Part model, mm, in its own coordinate system. A direction names the side the tool comes from. Coordinates: 2 decimals unless noted, no trailing zeros. Write each loop counter-clockwise with the first axis right and the second up, starting at its lowest first coordinate (ties: lowest second). Pieces come first, ordered by that corner, then holes. Notation, with made-up numbers: M 83.5,-4.75 L 116.5,-4.75 A20 ccw 116.5,17.25 Z; hole C 53.5,68 d2. An arc over 180 degrees is marked long. Use a Markdown table: item, result. Add a question column.
Q1. Wall check: L1, parallel to Y at x = -19, z = 4.5; L2, parallel to X at y = 15, z = 13; L3, parallel to X at y = -6.5, z = 1.25. Give the ranges that are in metal, low to high. Write a range as from..to.
Q2. Slice it at C-C on y = 5.5. Write the cut outline in (x, z), then the cut area to 3 significant figures.
Q3. Slice it at A-A on z = 12.5. Write the cut outline in (x, y).
Q4. Slice it at D-D on z = 3. Write the cut outline in (x, y).
Q5. Pin check, flat tips, straight feed: pin 1 Ø11 at (x, z) = (-0.5, 16) entering from +Y; pin 2 Ø1.5 at (y, z) = (13.5, 13.5) entering from -X; pin 3 Ø0.6 at (x, z) = (-7.5, 23) entering from -Y. Stop position of each tip, or through.
Q6. Slice it at B-B on x = 2. Write the cut outline in (y, z), then the cut area to 3 significant figures.
Q7. Tool access for faces 5 (the flat face through (-1, -10.25, 6)), 6 (the flat face through (-45.75, -6.9, 22.5)), 7 (the flat face through (41.75, 13, 11)), 8 (the flat face through (-8, 12.25, 13)): list every direction of +Z, -Z, +X, -X, +Y, -Y with a clear straight run to the whole face (end or side of a thin tool).
Q8. Mould opens along Y. For faces 1 (the flat face through (-5, 10.25, 11)), 2 (the flat face through (38.75, 13, 11)), 3 (the flat face through (22, 17.25, 1)), 4 (the flat face through (-2, 7.25, 23)) say: released by +Y, released by -Y, zero draft, split by the parting line, or undercut.
from build123d import *

# Parameters (mm, degrees)
EXTRUDE_1_DEPTH          = 8
EXTRUDE_3_DEPTH          = 14
CUT_EXTRUDE_1_DEPTH      = 55.485089704
CUT_EXTRUDE_1_DEPTH_BACK = 55.485089704
SKETCH_4_W               = 2
SKETCH_4_H               = 24.5
SKETCH_7_W               = 2
SKETCH_7_H               = 2
SKETCH_7_W_2             = 5
EXTRUDE_6_DEPTH          = 14
EXTRUDE_4_DEPTH          = 2
SKETCH_8_W               = 85.5
SKETCH_8_H               = 1.5
EXTRUDE_7_DEPTH          = 5


with BuildPart() as part:
    # Эскиз1 → Бобышка-Вытянуть1 (new body)
    with BuildSketch(Plane.XY):
        Polygon((47.75, 12.25), (44.75, 12.25), (44.75, 17.25), (35.75, 17.25), (35.75, 12.25), (-49.75, 12.25), (-49.75, -12.25), (47.75, -12.25), (47.75, -10.25), (-47.75, -10.25), (-47.75, 10.25), (38.75, 10.25), (38.75, 15.25), (41.75, 15.25), (41.75, 12.25), (41.75, 10.25), (47.75, 10.25), align=None)
    extrude(amount=EXTRUDE_1_DEPTH)

    # Эскиз2 → Бобышка-Вытянуть3 (add)
    with BuildSketch(Plane.XY.offset(8)):
        Polygon((44.75, 10.25), (47.75, 10.25), (47.75, 12.25), (44.75, 12.25), (44.75, 15.25), (44.75, 17.25), (41.75, 17.25), (35.75, 17.25), (35.75, 15.25), (35.75, 12.25), (-47.75, 12.25), (-49.75, 12.25), (-49.75, 10.25), (-49.75, -10.25), (-49.75, -12.25), (-47.75, -12.25), (-47.75, -10.25), (-47.75, 10.25), (35.75, 10.25), (38.75, 10.25), (38.75, 12.25), (38.75, 15.25), (41.75, 15.25), (41.75, 10.25), align=None)
    extrude(amount=EXTRUDE_3_DEPTH)

    # Эскиз4 → Вырез-Вытянуть1 (cut, two sides: drawn at the far end of the back side and taken through both)
    with BuildSketch(Plane.XY.offset(8).offset(-CUT_EXTRUDE_1_DEPTH_BACK)):
        with Locations((46.75, 0)):
            Rectangle(SKETCH_4_W, SKETCH_4_H)
    extrude(amount=CUT_EXTRUDE_1_DEPTH + CUT_EXTRUDE_1_DEPTH_BACK, mode=Mode.SUBTRACT)

    # Эскиз7 → Бобышка-Вытянуть6 (add)
    with BuildSketch(Plane.XY.offset(8)):
        with Locations((-46.75, -11.25)):
            Rectangle(SKETCH_7_W, SKETCH_7_H)
        with Locations((43.25, -11.25)):
            Rectangle(SKETCH_7_W_2, SKETCH_7_H)
    extrude(amount=EXTRUDE_6_DEPTH)

    # Эскиз5 → Бобышка-Вытянуть4 (add)
    with BuildSketch(Plane.XY.offset(22)):
        Polygon((45.75, -12.25), (40.75, -12.25), (40.75, 7.25), (-45.75, 7.25), (-45.75, -12.25), (-49.75, -12.25), (-49.75, 12.25), (35.75, 12.25), (35.75, 17.25), (44.75, 17.25), (44.75, 12.25), (45.75, 12.25), align=None)
    extrude(amount=EXTRUDE_4_DEPTH)

    # Эскиз8 → Бобышка-Вытянуть7 (add)
    with BuildSketch(Plane(origin=(0, 12.25, 0), x_dir=(1, 0, 0), z_dir=(0, 1, 0))):
        with Locations((-7, -0.75)):
            Rectangle(SKETCH_8_W, SKETCH_8_H)
    extrude(amount=EXTRUDE_7_DEPTH)


solid = part.part
Recorded:
| question | item | result |
|---|---|---|
| 1 | L1 | -12.25..-10.25, 10.25..12.25 |
| 1 | L2 | 35.75..38.75, 41.75..44.75 |
| 1 | L3 | -49.75..-47.75 |
| 2 | outline | M -49.75,0 L -47.75,0 L -47.75,22 L -45.75,22 L -45.75,24 L -49.75,24 Z; M 40.75,22 L 45.75,22 L 45.75,24 L 40.75,24 Z |
| 2 | area | 62.0 mm² |
| 3 | outline | M -49.75,-12.25 L -45.75,-12.25 L -45.75,-10.25 L -47.75,-10.25 L -47.75,10.25 L 38.75,10.25 L 38.75,15.25 L 41.75,15.25 L 41.75,10.25 L 45.75,10.25 L 45.75,12.25 L 44.75,12.25 L 44.75,17.25 L 35.75,17.25 L 35.75,12.25 L -49.75,12.25 Z; M 40.75,-12.25 L 45.75,-12.25 L 45.75,-10.25 L 40.75,-10.25 Z |
| 4 | outline | M -49.75,-12.25 L 45.75,-12.25 L 45.75,-10.25 L -47.75,-10.25 L -47.75,10.25 L 38.75,10.25 L 38.75,15.25 L 41.75,15.25 L 41.75,10.25 L 45.75,10.25 L 45.75,12.25 L 44.75,12.25 L 44.75,17.25 L 35.75,17.25 L 35.75,12.25 L -49.75,12.25 Z |
| 5 | pin 1 | y = 12.25 |
| 5 | pin 2 | x = 35.75 |
| 5 | pin 3 | y = 7.25 |
| 6 | outline | M -12.25,0 L -10.25,0 L -10.25,8 L -12.25,8 Z; M 7.25,22 L 10.25,22 L 10.25,0 L 17.25,0 L 17.25,1.5 L 12.25,1.5 L 12.25,24 L 7.25,24 Z |
| 6 | area | 77.5 mm² |
| 7 | face 5 | -Z, +X |
| 7 | face 6 | +Z, -Y |
| 7 | face 7 | -Z |
| 7 | face 8 | +Z, -X, +Y |
| 8 | face 1 | undercut |
| 8 | face 2 | undercut |
| 8 | face 3 | released by +Y |
| 8 | face 4 | released by -Y |
